Geometry: final body of the model. Coordinates: model frame, mm. Round coordinates to 2 decimals unless told otherwise and drop trailing zeros. Loops run counter-clockwise (first coordinate to the right, second up) from the corner with the lowest first, then second, coordinate; pieces in that order, holes last. Notation, with made-up numbers: M 22,29 L 29,29 A7 ccw 29,41 Z; hole C -8.75,54.5 d2. An arc over 180 degrees is marked long. Answer as a JSON object with one key per item and string values.
Autodesk Inventor part; units mm, degrees
ref_plane "YZ Plane" through (0, 0, 0) normal (1, 0, 0) x (0, 1, 0)
ref_plane "XZ Plane" through (0, 0, 0) normal (0, 1, 0) x (-1, 0, 0)
ref_plane "XY Plane" through (0, 0, 0) normal (0, 0, 1) x (1, 0, 0)
sketch "草图1" plane through (0, 0, 0) normal (0, 0, 1) x (1, 0, 0)
  circle A0 centre (0, 0) radius 2.5
  line L0 (2.3094, -4) -> (-2.3094, -4)
  line L1 (-2.3094, -4) -> (-4.6188, 0)
  line L2 (-4.6188, 0) -> (-2.3094, 4)
  line L3 (-2.3094, 4) -> (2.3094, 4)
  line L4 (2.3094, 4) -> (4.6188, 0)
  line L5 (4.6188, 0) -> (2.3094, -4)
  line L6 (0, 0) -> (0, 1.5398)
  point P0 (0, 4)
  dimension "d0" = 5
  dimension "d1" = 1.5398
  dimension "d2" = 8
extrude "拉伸1" add sketch "草图1" along normal blind 5
thread "螺纹1"
fillet "圆角1" radius 0.25 12 edges at (0, 4, 5) (3.4641, 2, 5) (3.4641, -2, 5) (-3.4641, -2, 5) (-3.4641, 2, 5) (0, -4, 5) (3.4641, -2, 0) (3.4641, 2, 0) (0, 4, 0) (-3.4641, 2, 0) (-3.4641, -2, 0) (0, -4, 0)
chamfer "倒角1" distance 0.25 angle 45 2 edges at (-2.5, 0, 5) (-2.5, 0, 0)
properties part number "砂轮架带动曲柄轴盖螺帽"
1) Ray query, line 1 (Y direction, x = 0, z = 2.2); line 2 (Y direction, x = -1, z = 2.7); line 3 (X direction, y = 0.5, z = 1). Return the intervals inside material, ascending.
Results:
{"line 1": "-4 to -2.5, 2.5 to 4", "line 2": "-4 to -2.29, 2.29 to 4", "line 3": "-4.33 to -2.45, 2.45 to 4.33"}
2) Pull-direction query (X, two-part tool) for faces 1 (the cylindrical face through (-0.54, 2.44, 2.47)), 2 (the cylindrical face through (3.42, 1.94, 4.92)), 3 (the cylindrical face through (-3.415, -1.934, 0.071)); classes: +X half, -X half, draft (parallel to the pull), parting line (faces both ways), or undercut.
Results:
{"face 1": "undercut", "face 2": "+X half", "face 3": "-X half"}
3) Section query B-B (x = 0). Return the cut outline in (y, z).
Results:
{"outline": "M -4,0.25 A0.25 ccw -3.75,0 L -2.75,0 L -2.5,0.25 L -2.5,4.75 L -2.75,5 L -3.75,5 A0.25 ccw -4,4.75 Z; M 2.5,0.25 L 2.75,0 L 3.75,0 A0.25 ccw 4,0.25 L 4,4.75 A0.25 ccw 3.75,5 L 2.75,5 L 2.5,4.75 Z"}
4) Section query A-A (z = 2.1). Return the cut outline in (x, y).
Results:
{"outline": "M -4.62,0 L -2.31,-4 L 2.31,-4 L 4.62,0 L 2.31,4 L -2.31,4 Z; hole C 0,0 d5"}
5) Pin query (flat end, axial travel): P1, Ø4, axis at x = 0, y = 0, coming from the -Z side; P2, Ø3, axis at y = 2, z = 3.5, coming from the +X side. Return the tip coordinate at first contact, or that it passes through.
Results:
{"P1": "through", "P2": "x = 4.33"}
